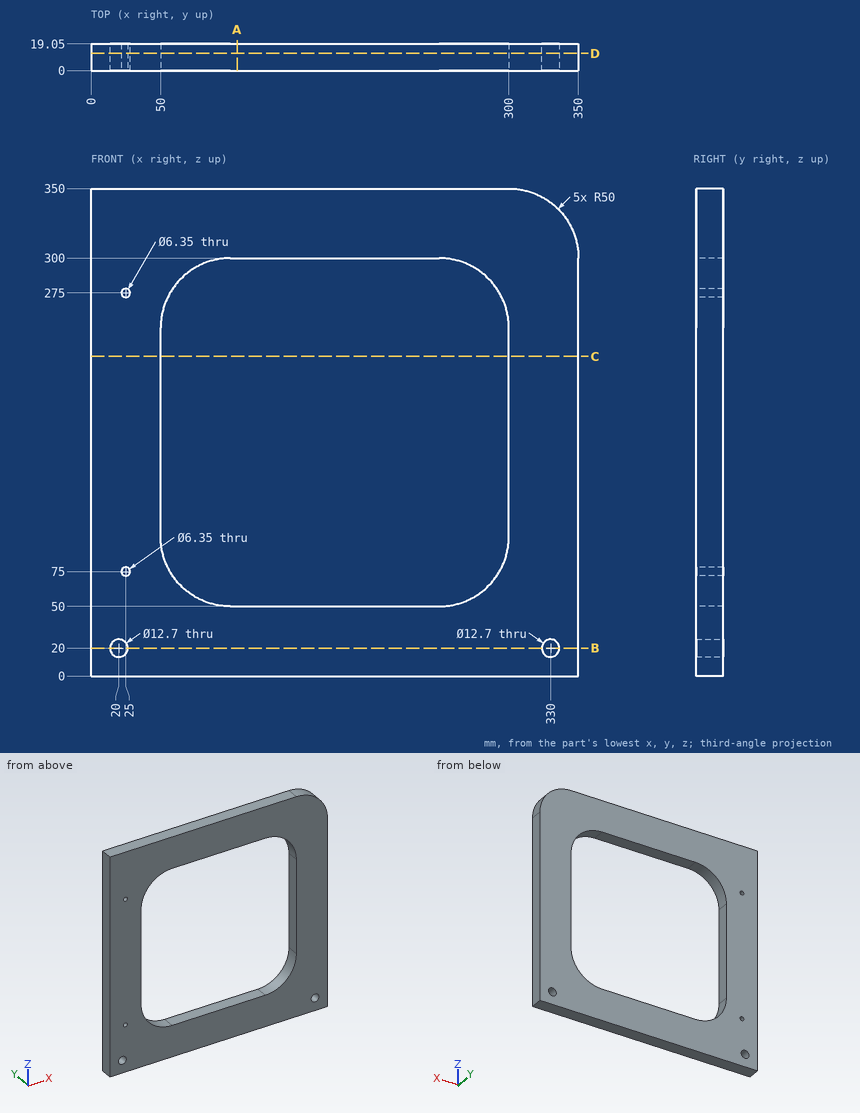
Job drawing, mm, ordinate dimensions from the low corner. One solid piece. Round coordinates to 2 decimals unless told otherwise and drop trailing zeros. Loops run counter-clockwise (first coordinate to the right, second up) from the corner with the lowest first, then second, coordinate; pieces in that order, holes last.
(1) Cut at B-B (z = 20). Give the cut face in (x, y).
(2) Cut at C-C (z = 229.5). Give the cut face in (x, y).
(3) Cut at D-D (y = 12.25). Give the cut face in (x, z) (3 decimals), plus the area to 3 significant figures.
(4) Cut at A-A (x = 105). Give the cut face in (y, z).
(5) Wall check: line 1 along X through (y, z) = (15.75, 245.5); line 2 along Z through (x, y) = (20, 8.75). Give the ranges that are in metal, low to high.
Findings below:
1. outline: (0, 0) - (13.65, 0) - (13.65, 19.05) - (0, 19.05) - close; (26.35, 0) - (323.65, 0) - (323.65, 19.05) - (26.35, 19.05) - close; (336.35, 0) - (350, 0) - (350, 19.05) - (336.35, 19.05) - close
2. outline: (0, 0) - (50, 0) - (50, 19.05) - (0, 19.05) - close; (300, 0) - (350, 0) - (350, 19.05) - (300, 19.05) - close
3. outline: (0, 0) - (350, 0) - (350, 300) arc R50 ccw to (300, 350) - (0, 350) - close; hole circle Ø12.7 at (20, 20); hole circle Ø6.35 at (25, 75); hole circle Ø6.35 at (25, 275); hole (50, 100) arc R50 ccw to (100, 50) - (250, 50) arc R50 ccw to (300, 100) - (300, 250) arc R50 ccw to (250, 300) - (100, 300) arc R50 ccw to (50, 250) - close; hole circle Ø12.7 at (330, 20)
3. area: 61,300 mm2
4. outline: (0, 0) - (19.05, 0) - (19.05, 50) - (0, 50) - close; (0, 300) - (19.05, 300) - (19.05, 350) - (0, 350) - close
5. line 1: x = 0 to 50, 300 to 350
5. line 2: z = 0 to 13.65, 26.35 to 350
